Could you check a few things on this model? Use its own coordinates, in mm. Face numbers are marked on the shaded views. Round coordinates to 2 decimals unless told otherwise and drop trailing zeros. Order: outer loops, then holes, each group sorted by start corner. A loop starts at its lowest first (then second) coordinate and runs counter-clockwise, first axis right, second up. Notation, with made-up numbers: (43, 43) - (72, 43) arc R27 ccw to (72, 82) - close; hole circle Ø1 at (-18, -33.5). An arc over 180 degrees is marked (long way). Use one line per item in the form item = value.
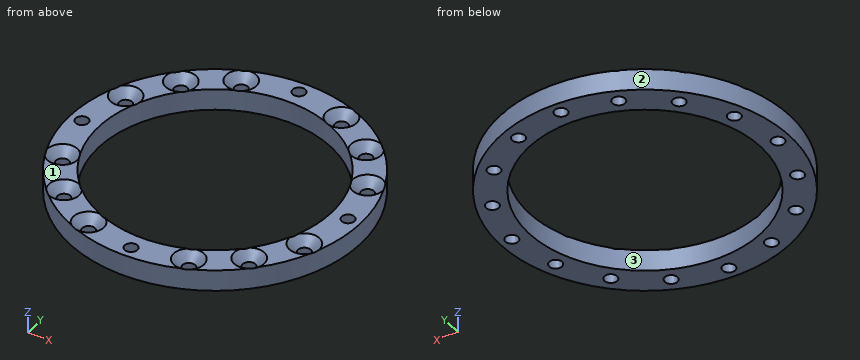
from build123d import *

# Parameters (mm, degrees)
ESQUISSE1_R             = 37.5
ESQUISSE1_R_2           = 30
BOSS_EXTRU_1_DEPTH      = 5.5
ESQUISSE2_R             = 1.65
ENL_V_MAT_EXTRU_1_DEPTH = 54.31744555
CHANFREIN1_SIZE         = 2.25


with BuildPart() as part:
    # Esquisse1 → Boss.-Extru.1 (new body)
    with BuildSketch(Plane.XY):
        Circle(ESQUISSE1_R)
        Circle(ESQUISSE1_R_2, mode=Mode.SUBTRACT)
    extrude(amount=BOSS_EXTRU_1_DEPTH)

    # Esquisse2 → Enlèv. mat.-Extru.1 (cut, through all)
    with BuildSketch(Plane.XY.offset(5.5)):
        with Locations((0, 34.3)):
            Circle(ESQUISSE2_R)
        with Locations((12.915565842, 31.180934222)):
            Circle(ESQUISSE2_R)
        with Locations((23.864853865, 23.864853865)):
            Circle(ESQUISSE2_R)
        with Locations((31.180934222, 12.915565842)):
            Circle(ESQUISSE2_R)
        with Locations((34.3, 0)):
            Circle(ESQUISSE2_R)
        with Locations((31.180934222, -12.915565842)):
            Circle(ESQUISSE2_R)
        with Locations((23.864853865, -23.864853865)):
            Circle(ESQUISSE2_R)
        with Locations((12.915565842, -31.180934222)):
            Circle(ESQUISSE2_R)
        with Locations((0, -34.3)):
            Circle(ESQUISSE2_R)
        with Locations((-12.915565842, -31.180934222)):
            Circle(ESQUISSE2_R)
        with Locations((-23.864853865, -23.864853865)):
            Circle(ESQUISSE2_R)
        with Locations((-31.180934222, -12.915565842)):
            Circle(ESQUISSE2_R)
        with Locations((-34.3, 0)):
            Circle(ESQUISSE2_R)
        with Locations((-31.180934222, 12.915565842)):
            Circle(ESQUISSE2_R)
        with Locations((-23.864853865, 23.864853865)):
            Circle(ESQUISSE2_R)
        with Locations((-12.915565842, 31.180934222)):
            Circle(ESQUISSE2_R)
    extrude(amount=-ENL_V_MAT_EXTRU_1_DEPTH, mode=Mode.SUBTRACT)

    # Chanfrein1
    # the kernel refuses this chamfer: 2.25 mm, written as the material it takes off along each edge
    with BuildSketch(Plane(origin=(-12.915565842, 31.180934222, 5.5), x_dir=(1, 0, 0), z_dir=(0, -1, 0))) as chanfrein1_piece_1:
        Polygon((1.65 + CHANFREIN1_SIZE, 0), (1.65, -CHANFREIN1_SIZE), (1.65, 0), align=None)
    revolve(axis=Axis((-12.915565842, 31.180934222, 5.5), (0, 0, 1)), mode=Mode.SUBTRACT)
    with BuildSketch(Plane(origin=(-23.864853865, 23.864853865, 5.5), x_dir=(1, 0, 0), z_dir=(0, -1, 0))) as chanfrein1_piece_2:
        Polygon((1.65 + CHANFREIN1_SIZE, 0), (1.65, -CHANFREIN1_SIZE), (1.65, 0), align=None)
    revolve(axis=Axis((-23.864853865, 23.864853865, 5.5), (0, 0, 1)), mode=Mode.SUBTRACT)
    with BuildSketch(Plane(origin=(-31.180934222, 12.915565842, 5.5), x_dir=(1, 0, 0), z_dir=(0, -1, 0))) as chanfrein1_piece_3:
        Polygon((1.65 + CHANFREIN1_SIZE, 0), (1.65, -CHANFREIN1_SIZE), (1.65, 0), align=None)
    revolve(axis=Axis((-31.180934222, 12.915565842, 5.5), (0, 0, 1)), mode=Mode.SUBTRACT)
    with BuildSketch(Plane(origin=(-31.180934222, -12.915565842, 5.5), x_dir=(1, 0, 0), z_dir=(0, -1, 0))) as chanfrein1_piece_4:
        Polygon((1.65 + CHANFREIN1_SIZE, 0), (1.65, -CHANFREIN1_SIZE), (1.65, 0), align=None)
    revolve(axis=Axis((-31.180934222, -12.915565842, 5.5), (0, 0, 1)), mode=Mode.SUBTRACT)
    with BuildSketch(Plane(origin=(-23.864853865, -23.864853865, 5.5), x_dir=(1, 0, 0), z_dir=(0, -1, 0))) as chanfrein1_piece_5:
        Polygon((1.65 + CHANFREIN1_SIZE, 0), (1.65, -CHANFREIN1_SIZE), (1.65, 0), align=None)
    revolve(axis=Axis((-23.864853865, -23.864853865, 5.5), (0, 0, 1)), mode=Mode.SUBTRACT)
    with BuildSketch(Plane(origin=(-12.915565842, -31.180934222, 5.5), x_dir=(1, 0, 0), z_dir=(0, -1, 0))) as chanfrein1_piece_6:
        Polygon((1.65 + CHANFREIN1_SIZE, 0), (1.65, -CHANFREIN1_SIZE), (1.65, 0), align=None)
    revolve(axis=Axis((-12.915565842, -31.180934222, 5.5), (0, 0, 1)), mode=Mode.SUBTRACT)
    with BuildSketch(Plane(origin=(12.915565842, -31.180934222, 5.5), x_dir=(1, 0, 0), z_dir=(0, -1, 0))) as chanfrein1_piece_7:
        Polygon((1.65 + CHANFREIN1_SIZE, 0), (1.65, -CHANFREIN1_SIZE), (1.65, 0), align=None)
    revolve(axis=Axis((12.915565842, -31.180934222, 5.5), (0, 0, 1)), mode=Mode.SUBTRACT)
    with BuildSketch(Plane(origin=(23.864853865, -23.864853865, 5.5), x_dir=(1, 0, 0), z_dir=(0, -1, 0))) as chanfrein1_piece_8:
        Polygon((1.65 + CHANFREIN1_SIZE, 0), (1.65, -CHANFREIN1_SIZE), (1.65, 0), align=None)
    revolve(axis=Axis((23.864853865, -23.864853865, 5.5), (0, 0, 1)), mode=Mode.SUBTRACT)
    with BuildSketch(Plane(origin=(31.180934222, -12.915565842, 5.5), x_dir=(1, 0, 0), z_dir=(0, -1, 0))) as chanfrein1_piece_9:
        Polygon((1.65 + CHANFREIN1_SIZE, 0), (1.65, -CHANFREIN1_SIZE), (1.65, 0), align=None)
    revolve(axis=Axis((31.180934222, -12.915565842, 5.5), (0, 0, 1)), mode=Mode.SUBTRACT)
    with BuildSketch(Plane(origin=(31.180934222, 12.915565842, 5.5), x_dir=(1, 0, 0), z_dir=(0, -1, 0))) as chanfrein1_piece_10:
        Polygon((1.65 + CHANFREIN1_SIZE, 0), (1.65, -CHANFREIN1_SIZE), (1.65, 0), align=None)
    revolve(axis=Axis((31.180934222, 12.915565842, 5.5), (0, 0, 1)), mode=Mode.SUBTRACT)
    with BuildSketch(Plane(origin=(23.864853865, 23.864853865, 5.5), x_dir=(1, 0, 0), z_dir=(0, -1, 0))) as chanfrein1_piece_11:
        Polygon((1.65 + CHANFREIN1_SIZE, 0), (1.65, -CHANFREIN1_SIZE), (1.65, 0), align=None)
    revolve(axis=Axis((23.864853865, 23.864853865, 5.5), (0, 0, 1)), mode=Mode.SUBTRACT)
    with BuildSketch(Plane(origin=(12.915565842, 31.180934222, 5.5), x_dir=(1, 0, 0), z_dir=(0, -1, 0))) as chanfrein1_piece_12:
        Polygon((1.65 + CHANFREIN1_SIZE, 0), (1.65, -CHANFREIN1_SIZE), (1.65, 0), align=None)
    revolve(axis=Axis((12.915565842, 31.180934222, 5.5), (0, 0, 1)), mode=Mode.SUBTRACT)


solid = part.part
Item 1: If we mould it in two halves opening along X, with no side actions, what happens to the marked faces 1, 2 and 3? For each: released by +X, released by -X, zero draft, split by the parting line, or undercut.
Found:
face_1 = zero draft
face_2 = split by the parting line
face_3 = undercut
Item 2: Imagine slicing it at D-D on z = 1.5. State how many separate pieces and enclosed holes the cut face has, plus the area to 3 significant figures.
Found:
separate_pieces = 1
enclosed_holes = 17
area = 1,450 mm2
Item 3: Imagine slicing it at A-A on y = 0. Please give me the cut outline in (x, z).
Found:
outline = (-37.5, 0) - (-35.95, 0) - (-35.95, 5.5) - (-37.5, 5.5) - close; (-32.65, 0) - (-30, 0) - (-30, 5.5) - (-32.65, 5.5) - close; (30, 0) - (32.65, 0) - (32.65, 5.5) - (30, 5.5) - close; (35.95, 0) - (37.5, 0) - (37.5, 5.5) - (35.95, 5.5) - close
Item 4: I need wall thicknesses on L1, parallel to Y at x = 0, z = 2.25; L2, parallel to Y at x = 23, z = 4.65; L3, parallel to Y at x = 33.5, z = 1.3. Which ranges of each line are inside material? Lowest first, please.
Found:
L1 = -37.5 to -35.95, -32.65 to -30, 30 to 32.65, 35.95 to 37.5
L2 = -29.62 to -26.79, -20.94 to -19.26, 19.26 to 20.94, 26.79 to 29.62
L3 = -16.85 to -1.44, 1.44 to 16.85
Item 5: Will these pins go through, and if not, where does the flat tip stop? P1, Ø4.5, axis at x = 12.92, y = -31.18, coming from the +Z side; P2, Ø1.5, axis at x = 9.5, z = 2.5, coming from the -Y side; P3, Ø1.5, axis at x = -28.5, z = 4.5, coming from the -Y side.
Found:
P1 = 3.85
P2 = -36.46
P3 = -25.22
Item 6: Imagine slicing it at C-C on x = 18.5. Please give me the cut outline in (y, z).
Found:
outline = (-32.62, 0) - (-23.62, 0) - (-23.62, 5.5) - (-32.62, 5.5) - close; (23.62, 0) - (32.62, 0) - (32.62, 5.5) - (23.62, 5.5) - close
